Check sheet for the modelled part. Datum: model origin and axes. Units: mm. A direction names the side the tool comes from. Round coordinates to 2 decimals unless told otherwise and drop trailing zeros. Loops run counter-clockwise (first coordinate to the right, second up) from the corner with the lowest first, then second, coordinate; pieces in that order, holes last. Notation, with made-up numbers: (73.25, -36.75) - (103.25, -36.75) arc R20 cw to (103.25, -32.75) - close; hole circle Ø11 at (47, 42). An arc over 180 degrees is marked (long way). Answer in a Markdown table with one row per item. Add a question column.
(1) Access from +Z, -Z, +X, -X, +Y, -Y to the whole of each face (thin tool, end or side, straight path). Record for faces 5 (the flat face through (27, -1, 1.5)), 6 (the flat face through (40, -1, 0)).
(2) Cross-section at B-B on x = -5. Enter the section's corners in (y, z), then the cut area to 3 significant figures.
(3) Mould release check, pull along X, two halves, no side actions. Record for faces 1 (the cylindrical face through (39.1, -0.76, 11.64)), 2 (the flat face through (26, -1, -1.5)), 3 (the flat face through (-40, -1, 0)), 4 (the cylindrical face through (17.5, -0.7, 0)): +X half, -X half, draft (parallel to the pull), parting line (faces both ways), or undercut.
(4) Cross-section at A-A on z = 0. Enter the section's corners in (x, y), then the cut area to 3 significant figures.
(5) Thickness scan on line 1 along Z through (x, y) = (-4.5, -0.15); line 2 along X through (y, z) = (-0.2, -9.75); line 3 along Z through (x, y) = (-30.5, -0.1). Record the ranges inside material, lowest first.
(6) Gauge pin test, flat end, axial feed: pin 1 (1.8 mm diameter, centred on x = -5, z = -8.66, fed in from +Y). Record the tip position at first contact, or that the pin passes through.
(7) Cross-section at C-C on y = -0.75. Enter the section's corners in (x, z).
from build123d import *

# Parameters (mm, degrees)
SKETCH2_W           = 80
SKETCH2_H           = 25
SKETCH2_R           = 1.5
BOSS_EXTRUDE1_DEPTH = 1.5
FILLET2_R           = 3


with BuildPart() as part:
    # Sketch2 → Boss-Extrude1 (new body)
    with BuildSketch(Plane(origin=(0, 0, 0), x_dir=(1, 0, 0), z_dir=(0, 1, 0))):
        Rectangle(SKETCH2_W, SKETCH2_H)
        with Locations(Location((5, -8.660254038, 0), (0, 0, 270))):
            Circle(SKETCH2_R, mode=Mode.SUBTRACT)
        with Locations(Location((-5, -8.660254038, 0), (0, 0, 270))):
            Circle(SKETCH2_R, mode=Mode.SUBTRACT)
        with Locations(Location((-5, 8.660254038, 0), (0, 0, 270))):
            Circle(SKETCH2_R, mode=Mode.SUBTRACT)
        with Locations(Location((5, 8.660254038, 0), (0, 0, 270))):
            Circle(SKETCH2_R, mode=Mode.SUBTRACT)
        with BuildLine():
            Line((34, -1.5), (19, -1.5))
            ThreePointArc((19, -1.5), (17.5, 0), (19, 1.5))
            Line((19, 1.5), (34, 1.5))
            ThreePointArc((34, 1.5), (35.5, 0), (34, -1.5))
        make_face(mode=Mode.SUBTRACT)
        with BuildLine():
            Line((-34, -1.5), (-19, -1.5))
            ThreePointArc((-19, -1.5), (-17.5, 0), (-19, 1.5))
            Line((-19, 1.5), (-34, 1.5))
            ThreePointArc((-34, 1.5), (-35.5, 0), (-34, -1.5))
        make_face(mode=Mode.SUBTRACT)
    extrude(amount=-BOSS_EXTRUDE1_DEPTH)

    # Fillet2
    fillet2_edges = [part.edges().sort_by_distance(p)[0] for p in [
        (40, -0.75, 12.5),
        (-40, -0.75, 12.5),
        (-40, -0.75, -12.5),
        (40, -0.75, -12.5),
    ]]
    fillet(fillet2_edges, radius=FILLET2_R)


solid = part.part
Answers:
| question | item | result |
|---|---|---|
| 1 | face 5 | +Y, -Y |
| 1 | face 6 | +Z, -Z, +X, +Y, -Y |
| 2 | outline | (-1.5, -12.5) - (0, -12.5) - (0, -10.16) - (-1.5, -10.16) - close; (-1.5, -7.16) - (0, -7.16) - (0, 7.16) - (-1.5, 7.16) - close; (-1.5, 10.16) - (0, 10.16) - (0, 12.5) - (-1.5, 12.5) - close |
| 2 | area | 28.5 mm^2 |
| 3 | face 1 | +X half |
| 3 | face 2 | undercut |
| 3 | face 3 | -X half |
| 3 | face 4 | undercut |
| 4 | outline | (-40, -1.5) - (-35.5, -1.5) - (-35.5, 0) - (-40, 0) - close; (-17.5, -1.5) - (17.5, -1.5) - (17.5, 0) - (-17.5, 0) - close; (35.5, -1.5) - (40, -1.5) - (40, 0) - (35.5, 0) - close |
| 4 | area | 66.0 mm^2 |
| 5 | line 1 | z = -12.5 to -10.07, -7.25 to 7.25, 10.07 to 12.5 |
| 5 | line 2 | x = -39.99 to -6.03, -3.97 to 3.97, 6.03 to 39.99 |
| 5 | line 3 | z = -12.5 to -1.5, 1.5 to 12.5 |
| 6 | pin 1 | passes through |
| 7 | outline | (-40, -9.5) arc R3 ccw to (-37, -12.5) - (37, -12.5) arc R3 ccw to (40, -9.5) - (40, 9.5) arc R3 ccw to (37, 12.5) - (-37, 12.5) arc R3 ccw to (-40, 9.5) - close; hole (-34, -1.5) - (-19, -1.5) arc R1.5 ccw to (-19, 1.5) - (-34, 1.5) arc R1.5 ccw to start; hole circle Ø3 at (-5, -8.66); hole circle Ø3 at (-5, 8.66); hole circle Ø3 at (5, -8.66); hole circle Ø3 at (5, 8.66); hole (19, -1.5) - (34, -1.5) arc R1.5 ccw to (34, 1.5) - (19, 1.5) arc R1.5 ccw to start |
